Verification items for the finished model (mm, model axes). Coordinates: 2 decimals unless noted, no trailing zeros. Loops run counter-clockwise (first coordinate to the right, second up) from the corner with the lowest first, then second, coordinate; pieces in that order, holes last. Notation, with made-up numbers: (38.25, 46.25) - (51.25, 46.25) arc R25 ccw to (51.25, 60.25) - close; hole circle Ø9 at (-8.75, 15.5). An arc over 180 degrees is marked (long way). Answer as CSV lines item,"result". Start each with the question number.
1. Gauge pin test, flat ends, axial feed: P1, Ø1.5, axis at y = 132.5, z = 1.5, coming from the +X side; P2, Ø2.5, axis at x = 128.875, y = 185, coming from the -Z side; P3, Ø0.9, axis at y = 211, z = 1, coming from the +X side; P4, Ø0.9, axis at y = 211, z = 1, coming from the -X side. Record the tip position at first contact, or that the pin passes through.
2. Material ranges on line 1 (X direction, y = 185, z = 1.4) (3 decimals); line 2 (Y direction, x = 129, z = 1.85); line 3 (Y direction, x = 110.5, z = 0.6), recorded low to high. Write a range as [from, to].
3. Cross-section at A-A (y = 108). Enter the section's corners in (x, z).
4. Cross-section at C-C (x = 74.5). Enter the section's corners in (y, z).
5. Cross-section at B-B (z = 1.15). State how many separate pieces and enclosed holes the cut face has, plus the area to 3 significant figures.
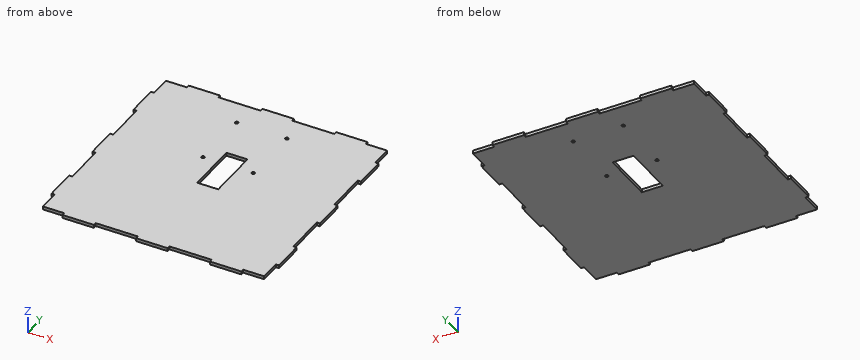
```python
from build123d import *

# Parameters (mm, degrees)
F0_R     = 1.5
F0_W     = 20
F0_H     = 50
F0_W_2   = 30
F0_H_2   = 3
F0_W_3   = 3
F0_H_3   = 30
F1_DEPTH = 3


with BuildPart() as f1:
    # F0 (on Top) → F1 (new body)
    with BuildSketch(Plane.XY):
        Polygon((0, 20), (0, 0), (20, 0), (50, 0), (90, 0), (120, 0), (160, 0), (190, 0), (210, 0), (210, 20), (210, 50), (210, 90), (210, 120), (210, 160), (210, 190), (210, 210), (190, 210), (160, 210), (120, 210), (90, 210), (50, 210), (20, 210), (0, 210), (0, 190), (0, 160), (0, 120), (0, 90), (0, 50), align=None)
        with Locations((81.125, 127.5)):
            Circle(F0_R, mode=Mode.SUBTRACT)
        with Locations((81.125, 185)):
            Circle(F0_R, mode=Mode.SUBTRACT)
        with Locations((105, 117.5)):
            Rectangle(F0_W, F0_H, mode=Mode.SUBTRACT)
        with Locations((128.875, 127.5)):
            Circle(F0_R, mode=Mode.SUBTRACT)
        with Locations((128.875, 185)):
            Circle(F0_R, mode=Mode.SUBTRACT)
        with Locations((35, -1.5)):
            Rectangle(F0_W_2, F0_H_2)
        with Locations((-1.5, 35)):
            Rectangle(F0_W_3, F0_H_3)
        with Locations((105, -1.5)):
            Rectangle(F0_W_2, F0_H_2)
        with Locations((-1.5, 105)):
            Rectangle(F0_W_3, F0_H_3)
        with Locations((175, -1.5)):
            Rectangle(F0_W_2, F0_H_2)
        with Locations((-1.5, 175)):
            Rectangle(F0_W_3, F0_H_3)
        with Locations((211.5, 35)):
            Rectangle(F0_W_3, F0_H_3)
        with Locations((35, 211.5)):
            Rectangle(F0_W_2, F0_H_2)
        with Locations((211.5, 105)):
            Rectangle(F0_W_3, F0_H_3)
        with Locations((105, 211.5)):
            Rectangle(F0_W_2, F0_H_2)
        with Locations((211.5, 175)):
            Rectangle(F0_W_3, F0_H_3)
        with Locations((175, 211.5)):
            Rectangle(F0_W_2, F0_H_2)
    extrude(amount=F1_DEPTH)


solid = f1.part
```
Values follow:
1,P1,"stops at x = 210"
1,P2,"passes through"
1,P3,"stops at x = 190"
1,P4,"stops at x = 20"
2,line 1,"x = [-3, 79.625], [82.625, 127.375], [130.375, 213]"
2,line 2,"y = [0, 126.01], [128.99, 183.51], [186.49, 210]"
2,line 3,"y = [-3, 92.5], [142.5, 213]"
3,outline,"(-3, 0) - (95, 0) - (95, 3) - (-3, 3) - close; (115, 0) - (213, 0) - (213, 3) - (115, 3) - close"
4,outline,"(0, 0) - (210, 0) - (210, 3) - (0, 3) - close"
5,separate pieces,"1"
5,enclosed holes,"5"
5,area,"44,200 mm²"
